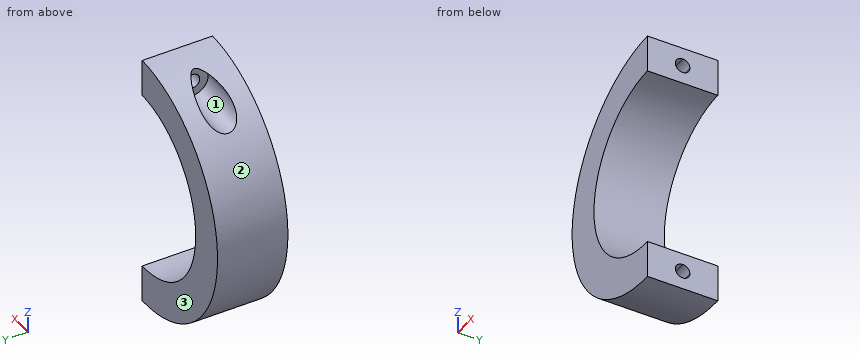
```python
from build123d import *

# Parameters (mm, degrees)
F1_DEPTH = 13.5
F3_DEPTH = 5
F4_R     = 3
F5_DEPTH = 25
F7_DEPTH = 7


with BuildPart() as f1:
    # F0 (on Front) → F1 (new body)
    with BuildSketch(Plane.XZ):
        with BuildLine():
            ThreePointArc((0, -17.75), (-17.75, 0), (0, 17.75))
            Line((0, 17.75), (0, 25))
            ThreePointArc((0, 25), (-25, 0), (0, -25))
            Line((0, -25), (0, -17.75))
        make_face()
    extrude(amount=F1_DEPTH)

    # F2 (on face) → F3 (cut)
    with BuildSketch(Plane.YZ):
        with BuildLine():
            ThreePointArc((-5.35, 21.375), (-5.760051, 22.364949), (-6.75, 22.775))
            Line((-6.75, 22.775), (-6.75, 19.975))
            ThreePointArc((-6.75, 19.975), (-5.760051, 20.385051), (-5.35, 21.375))
        make_face()
        with BuildLine():
            Line((-6.75, 19.975), (-6.75, 22.775))
            ThreePointArc((-6.75, 22.775), (-8.15, 21.375), (-6.75, 19.975))
        make_face()
    extrude(amount=-F3_DEPTH, mode=Mode.SUBTRACT)

    # F4 (on face) → F5 (cut)
    with BuildSketch(Plane.YZ.offset(-5)):
        with Locations((-6.75, 21.375)):
            Circle(F4_R)
    extrude(amount=-F5_DEPTH, mode=Mode.SUBTRACT)

    # F6 (on face) → F7 (cut)
    with BuildSketch(Plane.YZ):
        with BuildLine():
            ThreePointArc((-5.35, -21.375), (-5.760051, -20.385051), (-6.75, -19.975))
            Line((-6.75, -19.975), (-6.75, -22.775))
            ThreePointArc((-6.75, -22.775), (-5.760051, -22.364949), (-5.35, -21.375))
        make_face()
        with BuildLine():
            Line((-6.75, -22.775), (-6.75, -19.975))
            ThreePointArc((-6.75, -19.975), (-8.15, -21.375), (-6.75, -22.775))
        make_face()
    extrude(amount=-F7_DEPTH, mode=Mode.SUBTRACT)


solid = f1.part
```
Geometry check sheet. Reference: the model listing, model coordinates, mm. Face numbers are marked on the shaded views. Give positions to 0.01 mm unless a question says otherwise; leave off trailing zeros. Loops run counter-clockwise (first coordinate to the right, second up) from the corner with the lowest first, then second, coordinate; pieces in that order, holes last. Notation, with made-up numbers: M 10.5,-31 L 18.5,-31 A34 cw 18.5,6 Z; hole C 52.5,46.5 d1. An arc over 180 degrees is marked long. Answer as CSV lines item,"result".
Item 1: Material ranges on line 1 (Z direction, x = -9.25, y = -0.75); line 2 (Z direction, x = -7.75, y = -6.75) (3 decimals); line 3 (X direction, y = -3.25, z = 10) (3 decimals), recorded low to high.
Values:
line 1,"z = -23.23 to -15.15, 15.15 to 23.23"
line 2,"z = -23.768 to -15.969, 15.969 to 18.375"
line 3,"x = -22.913 to -14.665"
Item 2: Cross-section at A-A on x = -3.5. Count the separate pieces of the cut face and the enclosed holes in it, and give its area (3 significant figures).
Values:
separate pieces,"2"
enclosed holes,"2"
area,"186 mm²"
Item 3: Cross-section at C-C on z = 0. Record the cut outline in (x, y).
Values:
outline,"M -25,-13.5 L -17.75,-13.5 L -17.75,0 L -25,0 Z"
Item 4: Cross-section at B-B on y = -1. Record the cut outline in (x, z).
Values:
outline,"M 0,-25 L 0,-17.75 A17.75 cw 0,17.75 L 0,25 A25 ccw Z"
Item 5: Depth check by flat-ended pin: P1, Ø2, axis at x = -12, y = -3, coming from the -Z side; P2, Ø5, axis at x = -20, y = -7, coming from the -Z side; P3, Ø5, axis at y = -8, z = 20, coming from the -X side; P4, Ø2, axis at x = -19.5, z = 19.5, coming from the +Y side. Enter the tip coordinate at first touch or a pass-through.
Values:
P1,"stops at z = -22.45"
P2,"stops at z = -17.85"
P3,"stops at x = -17.85"
P4,"passes through"
Item 6: Release check for a two-part mould opening along Z. For the marked faces 1, 2 and 3 record: pulls with the +Z half, pulls with the -Z half, needs draft (parallel to the pull), parting line crosses it, or undercut.
Values:
face 1,"undercut"
face 2,"parting line crosses it"
face 3,"needs draft"
